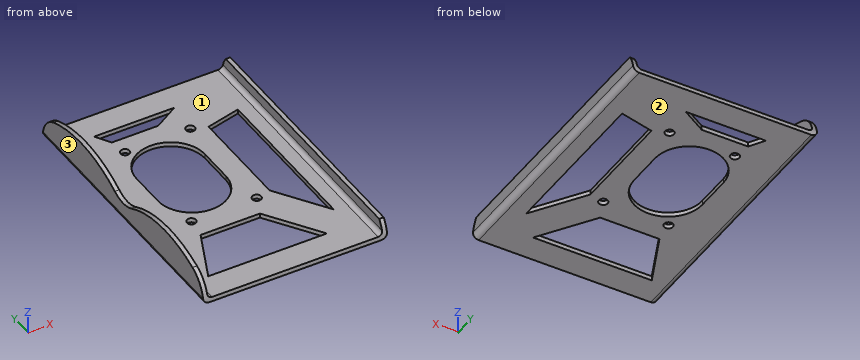
Autodesk Inventor part; units mm, degrees
ref_plane "YZ Plane" through (0, 0, 0) normal (1, 0, 0) x (0, 1, 0)
ref_plane "XZ Plane" through (0, 0, 0) normal (0, 1, 0) x (-1, 0, 0)
ref_plane "XY Plane" through (0, 0, 0) normal (0, 0, 1) x (1, 0, 0)
sketch "スケッチ1" plane through (0, 0, 0) normal (0, 0, 1) x (1, 0, 0)
  line L0 (-31, 46) -> (31, 46)
  line L1 (31, 46) -> (31, -46)
  line L2 (31, -46) -> (-31, -46)
  line L3 (-31, -46) -> (-31, 46)
  point P0 (0, 0)
  dimension "d0" = 92
  dimension "d1" = 46
  dimension "d2" = 62
  dimension "d3" = 31
extrude "押し出し1" add sketch "スケッチ1" along normal blind 1.5
sketch "スケッチ3" plane through (0, 0, 0) normal (0, 0, -1) x (-1, 0, 0)
  circle A0 centre (-7, 26) radius 1.5
  circle A1 centre (15, 26) radius 1.5
  circle A2 centre (-7, -12) radius 1.5
  circle A3 centre (15, -12) radius 1.5
  line L0 (31, 46) -> (-31, 46)
  line L1 (31, -46) -> (31, 46)
  point P0 (0, 0)
  dimension "d10" = 3
  dimension "d11" = 22
  dimension "d12" = 22
  dimension "d15" = 38
  dimension "d16" = 38
  dimension "d35" = 20
  dimension "d36" = 20
  dimension "d44" = 16
  dimension "d45" = 16
hole "穴1" at (-15, -12, 0) at (-15, 26, 0) at (7, 26, 0) at (7, -12, 0) direction (0, 0, 1) diameter 3 end through all
sketch "スケッチ4" plane through (0, 0, 1.5) normal (0, 0, 1) x (1, 0, 0)
  line L0 (-31, -46) -> (-31, 46)
  line L1 (31, -46) -> (-31, -46)
  line L2 (-31, 46) -> (-29.5, 46)
  line L3 (-29.5, 46) -> (-29.5, -46)
  line L4 (-29.5, -46) -> (-31, -46)
  line L5 (-31, -46) -> (-31, 46)
  line L6 (31, 46) -> (29.5, 46)
  line L7 (29.5, 46) -> (29.5, -46)
  line L8 (29.5, -46) -> (31, -46)
  line L9 (31, -46) -> (31, 46)
  point P0 (0, 0)
  dimension "d37" = 59
  dimension "d39" = 1.5
extrude "押し出し3" add sketch "スケッチ4" along normal blind 11
sketch "スケッチ5" plane through (-31, -46, 0) normal (-1, 0, 0) x (0, 0, 1)
  line L0 (0, 92) -> (12.5, 92)
  line L1 (0, 0) -> (0, 92)
  line L2 (0, 0) -> (12.5, 0)
  line L3 (12.5, 92) -> (12.5, 0)
  arc A0 (4.6931, 46) -> (6.25, 92) centre (-28.7857, 70.1595) ccw
  arc A1 (6.25, 0) -> (4.6931, 46) centre (-28.7857, 21.8405) ccw
  point P0 (0, 46)
extrude "押し出し4" cut sketch "スケッチ5" against normal blind 1.5 contours L0 L3 A0 | L3 A1 A0 | A1 L3 L2
sketch "スケッチ6" plane through (31, -46, 0) normal (1, 0, 0) x (0, 0, -1)
  line L0 (0, 0) -> (-12.5, 0)
  line L1 (-12.5, 92) -> (-6.25, 92)
  line L2 (-6.25, 92) -> (-6.25, 0)
  line L3 (-6.25, 0) -> (-12.5, 0)
  line L4 (-12.5, 0) -> (-12.5, 92)
  point P0 (0, 46)
extrude "押し出し5" cut sketch "スケッチ6" against normal blind 1.5
fillet "フィレット4" radius 10 3 edges at (-30.25, -46, 6.25) (-30.25, 0, 4.6931) (-30.25, 46, 6.25)
sketch "スケッチ7" plane through (0, 0, 1.5) normal (0, 0, 1) x (1, 0, 0)
  line L0 (-29.5, 45.9115) -> (29.5, 45.9115)
  line L1 (-29.5, 45.9115) -> (-29.5, -45.9115)
  line L2 (29.5, -45.9115) -> (-29.5, -45.9115)
  line L3 (29.5, -45.9115) -> (29.5, 45.9115)
  line L4 (4.5, 13.4115) -> (4.5, 1.4115)
  line L5 (-18.5, 1.4115) -> (-18.5, 13.4115)
  line L6 (-19, 36.9115) -> (8, 36.9115)
  line L7 (-0.3333, 31.9115) -> (-16, 31.9115)
  line L8 (-16, -18.9115) -> (4, -18.9115)
  line L9 (16, -36.9115) -> (-24, -36.9115)
  line L10 (-24, -36.9115) -> (-16, -18.9115)
  line L11 (16, -36.9115) -> (4, -18.9115)
  line L12 (31, 18.1628) -> (29.5, 17.5573)
  line L13 (-19, 36.9115) -> (-16, 31.9115)
  line L14 (8, 36.9115) -> (-0.3333, 31.9115)
  arc A0 (-18.5, 1.4115) -> (4.5, 1.4115) centre (-7, 1.4115) ccw
  arc A1 (4.5, 13.4115) -> (-18.5, 13.4115) centre (-7, 13.4115) ccw
  line L15 (-31, 39.7846) -> (-31, 4.7108)
  line L16 (-31, -4.7108) -> (-31, -39.7846)
  line L17 (31, 43.9415) -> (31, -43.9415)
  line L18 (12, -10.9115) -> (23.5, -28.1615)
  line L19 (23.5, -28.1615) -> (23.5, 26.8385)
  line L20 (23.5, 26.8385) -> (12, 24.0885)
  line L21 (12, -10.9115) -> (12, 24.0885)
  line L22 (29.5, -43.9415) -> (29.5, 43.9415)
  point P0 (0, 0)
  dimension "d62" = 12
  dimension "d63" = 11.5
  dimension "d64" = 11.5
  dimension "d65" = 23
  dimension "d68" = 32.5
  dimension "d70" = 5
  dimension "d72" = 18
  dimension "d73" = 27
  dimension "d77" = 9
  dimension "d78" = 13.5
  dimension "d79" = 10.5
  dimension "d80" = 11
  dimension "d83" = 24
  dimension "d84" = 24
  dimension "d89" = 40
  dimension "d92" = 20
  dimension "d93" = 9
  dimension "d102" = 7
  dimension "d103" = 15
  dimension "d114" = 35
  dimension "d115" = 55
  dimension "d118" = 11.5
  dimension "d119" = 6
  dimension "d120" = 35
extrude "押し出し6" cut sketch "スケッチ7" against normal blind 1.5 contours L4 A0 L5 A1 | L6 L14 L7 L13 | L8 L11 L9 L10 | L21 L20 L19 L18
fillet "フィレット5" radius 2 2 edges at (-31, 0, 0) (31, 0, 0)
fillet "フィレット5" radius 1.5 2 edges at (-29.5, 0, 1.5) (29.5, 0, 1.5)
properties material "アセタール樹脂、白"
Can you work these out from the model? Positions are in its coordinate system, mm. Face numbers are marked on the shaded views. Coordinates: 2 decimals unless noted, no trailing zeros. Write each loop counter-clockwise with the first axis right and the second up, starting at its lowest first coordinate (ties: lowest second). Pieces come first, ordered by that corner, then holes. Notation, with made-up numbers: M 9,17 L 34,17 A12 cw 34,37 Z; hole C 65,10 d2. An arc over 180 degrees is marked long. Write item = value, one per line. Start each with the question number.
Q1. If we section it at D-D, the plane x = -15: Write out the boundary of the cut face in (y, z).
Q2. If I drill on L1, parallel to X at y = 30.5, z = 4.5; L2, parallel to Y at x = -15, z = 0.75; L3, parallel to X at y = -12, z = 0.9, over which ranges is the centre line in solid material (lowest first)? Write a range as [from, to].
Q3. Thinking about a two-plate mould opening in X: for the marked faces 1, 2 and 3, which applies, released by +X, released by -X, zero draft, split by the parting line, or undercut?
Q4. If we section it at C-C, the plane z = 4.25: Write out the boundary of the cut face in (x, y).
Q5. If we section it at B-B, the plane y = 36: Write out the boundary of the cut face in (x, z), then the cut area to 3 significant figures.
Q6. If we section it at A-A, the plane x = -7: Write out the boundary of the cut face in (y, z), then the cut area to 3 significant figures.
Q7. I'm going to push flat-ended pins straight in: pin 1 (1.6 mm diameter, centred on y = 0.5, z = 0.5, fed in from +X); pin 2 (2.5 mm diameter, centred on x = 7, y = 26, fed in from -Z); pin 3 (2 mm diameter, centred on x = -13.5, y = -14.5, fed in from +Z); pin 4 (1.6 mm diameter, centred on x = 30, y = -6.5, fed in from +Z). Where does each tip first touch, or does it pass through?
Check sheet entries:
q1.outline = M -46,0 L -36.91,0 L -36.91,1.5 L -45.91,1.5 A10 ccw -46,0.17 Z; M -18.91,0 L -13.5,0 L -13.5,1.5 L -18.91,1.5 Z; M -10.5,0 L -6.85,0 L -6.85,1.5 L -10.5,1.5 Z; M 21.67,0 L 24.5,0 L 24.5,1.5 L 21.67,1.5 Z; M 27.5,0 L 31.91,0 L 31.91,1.5 L 27.5,1.5 Z; M 36.91,0 L 46,0 L 46,0.17 A10 ccw 45.91,1.5 L 36.91,1.5 Z
q2.L1 = [-31, -29.5], [29.5, 31]
q2.L2 = [-45.98, -36.91], [-18.91, -13.5], [-10.5, -6.85], [21.67, 24.5], [27.5, 31.91], [36.91, 45.98]
q2.L3 = [-30.67, -16.5], [-13.5, 5.5], [8.5, 12.73], [23.5, 30.67]
q3.face_1 = undercut
q3.face_2 = zero draft
q3.face_3 = released by -X
q4.outline = M -31,-45.13 L -29.5,-45.13 L -29.5,45.13 L -31,45.13 Z; M 29.5,-45.13 L 31,-45.13 L 31,45.13 L 29.5,45.13 Z
q5.outline = M -31,2 A2 ccw -29,0 L -18.45,0 L -18.45,1.5 L -28,1.5 A1.5 cw -29.5,3 L -29.5,10.77 L -31,10.77 Z; M 6.48,0 L 29,0 A2 ccw 31,2 L 31,6.25 L 29.5,6.25 L 29.5,3 A1.5 cw 28,1.5 L 6.48,1.5 Z
q5.area = 75.9 mm²
q6.outline = M -46,0 L -36.91,0 L -36.91,1.5 L -45.91,1.5 A10 ccw -46,0.17 Z; M -18.91,0 L -10.09,0 L -10.09,1.5 L -18.91,1.5 Z; M 24.91,0 L 31.91,0 L 31.91,1.5 L 24.91,1.5 Z; M 36.91,0 L 46,0 L 46,0.17 A10 ccw 45.91,1.5 L 36.91,1.5 Z
q6.area = 50.9 mm²
q7.pin_1 = 30.87
q7.pin_2 = through
q7.pin_3 = 1.5
q7.pin_4 = 6.25
